Here's how the part is built. I have some questions about the finished solid (model axes, mm). Face numbers are marked on the shaded views. A direction names the side the tool comes from. Coordinates: 2 decimals unless noted, no trailing zeros. Write each loop counter-clockwise with the first axis right and the second up, starting at its lowest first coordinate (ties: lowest second). Pieces come first, ordered by that corner, then holes. Notation, with made-up numbers: M 77,19.25 L 91,19.25 A16 cw 91,43.25 Z; hole C 71.25,18 d5. An arc over 180 degrees is marked long. Use a Markdown table: item, result.
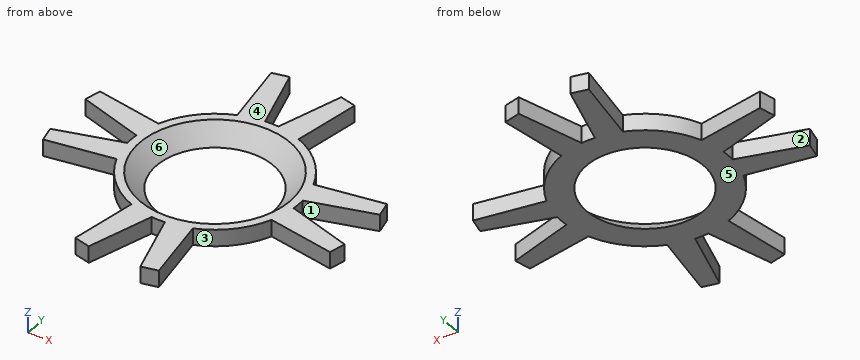
```python
from build123d import *

# Parameters (mm, degrees)
SKETCH_1_R              = 20
EXTRUDE_1_DEPTH         = 2
SKETCH_2_R              = 7
CUT_EXTRUDE_1_DEPTH     = 2
CUT_EXTRUDE_START       = -2
CUT_EXTRUDE_2_OUTLINE_R = 20
CUT_EXTRUDE_2_DEPTH     = 2
CHAMFER_4_SIZE          = 2


# Read off the part's stored shape, not the designer's step: 切除-拉伸2
with BuildPart() as part:
    # 草图1 → 凸台-拉伸1 (new body)
    with BuildSketch(Plane.XY):
        Circle(SKETCH_1_R)
    extrude(amount=EXTRUDE_1_DEPTH)

    # 草图2 → 切除-拉伸1 (cut)
    with BuildSketch(Plane.XY.offset(2)):
        Circle(SKETCH_2_R)
    extrude(amount=-CUT_EXTRUDE_1_DEPTH, mode=Mode.SUBTRACT)

    # 切除-拉伸2 outline → 切除-拉伸2 (cut)
    with BuildSketch(Plane.XY.offset(2).offset(CUT_EXTRUDE_START)):
        Circle(CUT_EXTRUDE_2_OUTLINE_R)
        with BuildLine():
            Line((-3.683674436, 9.296802819), (-5.007717322, 17.202301566))
            Line((-5.007717322, 17.202301566), (-3.091969732, 17.647553233))
            Line((-3.091969732, 17.647553233), (-0.793888425, 9.968437248))
            ThreePointArc((-0.793888425, 9.968437248), (0, 10), (0.793888425, 9.968437248))
            Line((0.793888425, 9.968437248), (3.091969732, 17.647553233))
            Line((3.091969732, 17.647553233), (5.007717322, 17.202301566))
            Line((5.007717322, 17.202301566), (3.683674436, 9.296802819))
            ThreePointArc((3.683674436, 9.296802819), (7.071067812, 7.071067812), (9.296802819, 3.683674436))
            Line((9.296802819, 3.683674436), (17.202301566, 5.007717322))
            Line((17.202301566, 5.007717322), (17.647553233, 3.091969732))
            Line((17.647553233, 3.091969732), (9.968437248, 0.793888425))
            ThreePointArc((9.968437248, 0.793888425), (10, 0), (9.968437248, -0.793888425))
            Line((9.968437248, -0.793888425), (17.647553233, -3.091969732))
            Line((17.647553233, -3.091969732), (17.202301566, -5.007717322))
            Line((17.202301566, -5.007717322), (9.296802819, -3.683674436))
            ThreePointArc((9.296802819, -3.683674436), (7.071067812, -7.071067812), (3.683674436, -9.296802819))
            Line((3.683674436, -9.296802819), (5.007717322, -17.202301566))
            Line((5.007717322, -17.202301566), (3.091969732, -17.647553233))
            Line((3.091969732, -17.647553233), (0.793888425, -9.968437248))
            ThreePointArc((0.793888425, -9.968437248), (0, -10), (-0.793888425, -9.968437248))
            Line((-0.793888425, -9.968437248), (-3.091969732, -17.647553233))
            Line((-3.091969732, -17.647553233), (-5.007717322, -17.202301566))
            Line((-5.007717322, -17.202301566), (-3.683674436, -9.296802819))
            ThreePointArc((-3.683674436, -9.296802819), (-7.071067812, -7.071067812), (-9.296802819, -3.683674436))
            Line((-9.296802819, -3.683674436), (-17.202301566, -5.007717322))
            Line((-17.202301566, -5.007717322), (-17.647553233, -3.091969732))
            Line((-17.647553233, -3.091969732), (-9.968437248, -0.793888425))
            ThreePointArc((-9.968437248, -0.793888425), (-10, 0), (-9.968437248, 0.793888425))
            Line((-9.968437248, 0.793888425), (-17.647553233, 3.091969732))
            Line((-17.647553233, 3.091969732), (-17.202301566, 5.007717322))
            Line((-17.202301566, 5.007717322), (-9.296802819, 3.683674436))
            ThreePointArc((-9.296802819, 3.683674436), (-7.071067812, 7.071067812), (-3.683674436, 9.296802819))
        make_face(mode=Mode.SUBTRACT)
    extrude(amount=CUT_EXTRUDE_2_DEPTH, mode=Mode.SUBTRACT)

    # 倒角4
    chamfer_4_edges = [part.edges().sort_by_distance(p)[0] for p in [
        (-7, 0, 2),
    ]]
    chamfer(chamfer_4_edges, length=CHAMFER_4_SIZE - 0.0001)  # a hair under: the kernel refuses the full size


solid = part.part
```
1. Suppose I cut it at D-D on x = -11. Write out the boundary of the cut face in (y, z).
Answers follow:
| item | result |
|---|---|
| outline | M -3.97,0 L -1.1,0 L -1.1,2 L -3.97,2 Z; M 1.1,0 L 3.97,0 L 3.97,2 L 1.1,2 Z |
2. Which directions (+Z, -Z, +X, -X, +Y, -Y) give clear straight access to the entire face, cutting with the end or side of a thin tool? Please do the marked faces 1, 2, 3 and 4.
Answers follow:
| item | result |
|---|---|
| face 1 | +Z, -Z, +X |
| face 2 | +Z, -Z, -X |
| face 3 | +Z, -Z |
| face 4 | +Z, +X, -X, +Y, -Y |
3. Will this pin go through, and if not, where does the flat tip stop? pin 1 Ø1.5 at (x, y) = (-2.5, 7.5) entering from -Z.
Answers follow:
| item | result |
|---|---|
| pin 1 | stops at z = 0 |
4. We'd pull the mould along Y, two halves only. Please class the marked faces 5 and 6: +Y half, -Y half, draft (parallel to the pull), parting line (faces both ways), or undercut.
Answers follow:
| item | result |
|---|---|
| face 5 | draft |
| face 6 | undercut |
5. I need wall thicknesses on probe 1 along X at (y, z) = (11.5, 1.9); probe 2 along Y at (x, z) = (-15, 1.25); probe 3 along X at (y, z) = (3.5, 1.15). Which ranges of each line are inside material? Lowest first, please.
Answers follow:
| item | result |
|---|---|
| probe 1 | x = -4.05 to -1.25, 1.25 to 4.05 |
| probe 2 | y = -4.64 to -2.3, 2.3 to 4.64 |
| probe 3 | x = -17.55 to -7.36, 7.36 to 17.55 |
